Work out the finished part from the listing and answer in its coordinate system (mm). A direction names the side the tool comes from. Give positions to 0.01 mm unless a question says otherwise; leave off trailing zeros. Loops run counter-clockwise (first coordinate to the right, second up) from the corner with the lowest first, then second, coordinate; pieces in that order, holes last. Notation, with made-up numbers: M 5,-23.5 L 14,-23.5 A26 cw 14,9.5 Z; hole C 54,-7.5 d7. An arc over 180 degrees is marked long. Answer in a Markdown table with one row per item. Add a question column.
from build123d import *

# Parameters (mm, degrees)
F2_DEPTH = 6.35
F3_R     = 3.81
F4_DEPTH = 25.4
F5_D     = 25.4


with BuildPart() as f2:
    # F1 (on Top) → F2 (new body)
    with BuildSketch(Plane.XY):
        with BuildLine():
            ThreePointArc((89.802561, -115.202561), (113.269101, -99.52272), (107.763073, -71.842049))
            Line((107.763073, -71.842049), (17.960512, 17.960512))
            ThreePointArc((17.960512, 17.960512), (0, 25.4), (-17.960512, 17.960512))
            Line((-17.960512, 17.960512), (-107.763073, -71.842049))
            ThreePointArc((-107.763073, -71.842049), (-113.269101, -99.52272), (-89.802561, -115.202561))
            Line((-89.802561, -115.202561), (89.802561, -115.202561))
        make_face()
    extrude(amount=F2_DEPTH)

    # F3 (on face) → F4 (join)
    with BuildSketch(Plane.XY.offset(6.35)):
        with Locations((89.802561, -89.802561)):
            Circle(F3_R)
        with Locations((-89.802561, -89.802561)):
            Circle(F3_R)
    extrude(amount=F4_DEPTH)

    # F5 (through all)
    with Locations(Plane(origin=(0, 0, 0), x_dir=(1, 0, 0), z_dir=(0, 0, -1))):
        with Locations((0, 0)):
            Hole(F5_D / 2)


solid = f2.part
(1) The mould has two halves that part along X. Classify faces 1 (the face through (-113.43, -99.13, 3.13)), 2 (the face through (113.106, -99.908, 3.131)), 3 (the face through (2.75, 12.4, 3.22)), 4 (the face through (-2, -60, 0)): pulls with the +X half, pulls with the -X half, needs draft (parallel to the pull), parting line crosses it, or undercut.
(2) Section D-D, the plane y = -100.5 is taken. Determine the outline of the cut face in (x, z), and give its area (3 significant figures).
(3) Which of the six approach directions +Z, -Z, +X, -X, +Y, -Y give full straight-line access (tool end or side, diameter ignored) to faces 5 (the face through (0.3, 25.4, 3.1)), 6 (the face through (-92.826, -92.121, 18.872))?
(4) Section B-B, the plane y = -2.5 is taken. Determine the outline of the cut face in (x, z), and give its area (3 significant figures).
(5) Section C-C, the plane z = 25 is taken. Determine the outline of the cut face in (x, y).
(6) Section A-A, the plane x = 0 is taken. Determine the outline of the cut face in (y, z).
(7) Consider line 1 along Y through (x, z) = (0, 3.5); line 2 along Z through (x, y) = (53, -42); line 3 along X through (y, z) = (-3, 2). Determine where each line is inside the solid, lowest interval first. Write a range as from..to.
(8) Each of these flat-tipped pins is pushed along its axis until it touches: P1, Ø6, axis at x = 50.5, y = -13, coming from the +Z side; P2, Ø1.5, axis at x = -37, y = -42, coming from the -Z side. Where does it stop, or does it pass through?
Numbers:
| question | item | result |
|---|---|---|
| 1 | face 1 | pulls with the -X half |
| 1 | face 2 | pulls with the +X half |
| 1 | face 3 | undercut |
| 1 | face 4 | needs draft |
| 2 | outline | M -112.84,0 L 112.84,0 L 112.84,6.35 L -112.84,6.35 Z |
| 2 | area | 1,430 mm² |
| 3 | face 5 | +Z, -Z, +Y |
| 3 | face 6 | +Z |
| 4 | outline | M -38.42,0 L -12.45,0 L -12.45,6.35 L -38.42,6.35 Z; M 12.45,0 L 38.42,0 L 38.42,6.35 L 12.45,6.35 Z |
| 4 | area | 330 mm² |
| 5 | outline | C -89.8,-89.8 d7.62; C 89.8,-89.8 d7.62 |
| 6 | outline | M -115.2,0 L -12.7,0 L -12.7,6.35 L -115.2,6.35 Z; M 12.7,0 L 25.4,0 L 25.4,6.35 L 12.7,6.35 Z |
| 7 | line 1 | y = -115.2..-12.7, 12.7..25.4 |
| 7 | line 2 | z = 0..6.35 |
| 7 | line 3 | x = -38.92..-12.34, 12.34..38.92 |
| 8 | P1 | stops at z = 6.35 |
| 8 | P2 | stops at z = 0 |
